Could you check a few things on this drawing? It's one solid part, dimensions in mm from its lowest x, y, z. A direction names the side the tool comes from. Coordinates: 2 decimals unless noted, no trailing zeros. Write each loop counter-clockwise with the first axis right and the second up, starting at its lowest first coordinate (ties: lowest second). Pieces come first, ordered by that corner, then holes.
Item 1: Please list where these lines run through material, in increasing order: line 1 (Z direction, x = 8, y = 6); line 2 (Z direction, x = 10.5, y = 13.25) (1 decimal); line 3 (X direction, y = 7, z = 25).
Item 2: I want a section at C-C (z = 44.5). Please give me the cut outline in (x, y).
Item 3: For the marked faces 1, 2 and 3, which set-ups out of +Z, -Z, +X, -X, +Y, -Y let a thin tool reach every point of the face, with its end or its side?
Item 4: If we mould it in two halves opening along Z, with no side actions, what happens to the marked faces 4, 5 and 6? For each: pulls with the +Z half, pulls with the -Z half, needs draft (parallel to the pull), parting line crosses it, or undercut.
Item 5: I want a section at B-B (y = 6.25). Please give me the cut outline in (x, z) (1 decimal), and give its area (4 significant figures).
Item 6: I'm going to push flat-ended pins straight in: P1, Ø1.5, axis at x = 10, z = 15.5, coming from the +Y side; P2, Ø10, axis at x = 16.5, y = 11, coming from the -Z side (1 decimal); P3, Ø10, axis at x = 9.5, z = 27, coming from the +Y side (1 decimal). Where does each tip first touch, or does it pass through?
Item 7: I want a section at D-D (x = 12). Please give me the cut outline in (y, z) (1 decimal), and give its area (3 significant figures).
Item 8: I want a section at A-A (x = 16.25). Please give me the cut outline in (y, z) (1 decimal).
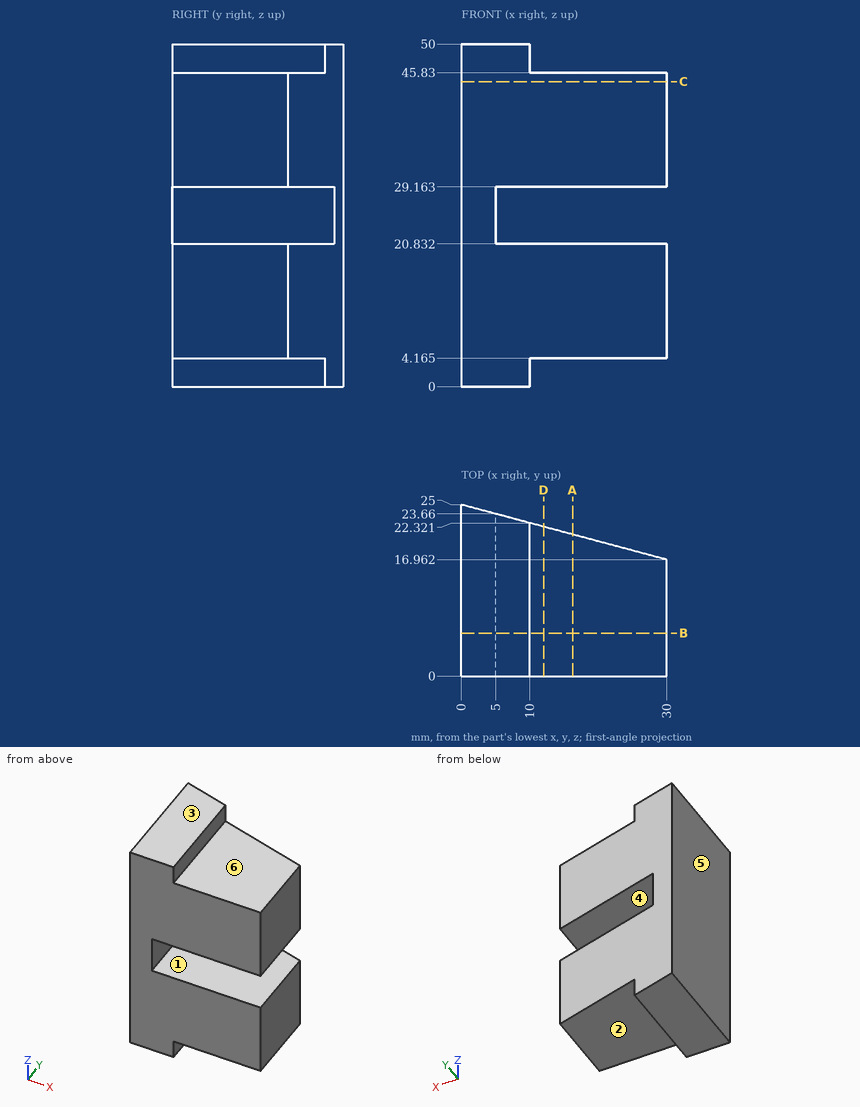
Answer:
1. line 1: z = 0 to 20.83, 29.16 to 50
1. line 2: z = 4.2 to 20.8, 29.2 to 45.8
1. line 3: x = 0 to 5
2. outline: (0, 0) - (30, 0) - (30, 16.96) - (0, 25) - close
3. face 1: +X, +Y, -Y
3. face 2: -Z, +X, +Y, -Y
3. face 3: +Z, +X, -X, +Y, -Y
4. face 4: undercut
4. face 5: needs draft
4. face 6: pulls with the +Z half
5. outline: (0, 0) - (10, 0) - (10, 4.2) - (30, 4.2) - (30, 20.8) - (5, 20.8) - (5, 29.2) - (30, 29.2) - (30, 45.8) - (10, 45.8) - (10, 50) - (0, 50) - close
5. area: 1,125 mm2
6. P1: stops at y = 22.52
6. P2: stops at z = 4.2
6. P3: stops at y = 23.8
7. outline: (0, 4.2) - (21.8, 4.2) - (21.8, 20.8) - (0, 20.8) - close; (0, 29.2) - (21.8, 29.2) - (21.8, 45.8) - (0, 45.8) - close
7. area: 726 mm2
8. outline: (0, 4.2) - (20.6, 4.2) - (20.6, 20.8) - (0, 20.8) - close; (0, 29.2) - (20.6, 29.2) - (20.6, 45.8) - (0, 45.8) - close
